Job drawing, mm, ordinate dimensions from the low corner. One solid piece. A direction names the side the tool comes from. Give positions to 0.01 mm unless a question says otherwise; leave off trailing zeros. Write each loop counter-clockwise with the first axis right and the second up, starting at its lowest first coordinate (ties: lowest second). Pieces come first, ordered by that corner, then holes. Notation, with made-up numbers: (7.25, -20) - (66.25, -20) arc R24 cw to (66.25, -8) - close; hole circle Ø3 at (55.5, -27). An arc over 180 degrees is marked (long way). Answer in a Markdown table with one row per item. Add a question column.
1. Band-saw the part on A-A on x = 8. Write the cut outline in (y, z), plus the area to 3 significant figures.
2. Probe line 1 along X through (y, z) = (95, 67); line 2 along Z through (x, y) = (52.5, 42); line 3 along Y through (x, z) = (47, 58). List the from-to ranges inside material, lowest first.
3. Band-saw the part on D-D on y = 95. Write the cut outline in (x, z), plus the area to 3 significant figures.
4. Which spindle directions (+Z, -Z, +X, -X, +Y, -Y) get a long thin tool onto all of the face, cutting with end or side? Do the marked faces 4, 5 and 6. Say none if no direction does.
5. Band-saw the part on C-C on x = 89. Write the cut outline in (y, z).
6. Drop flat-ended pins along their axis: pin 1 Ø1 at (x, z) = (46.5, 14) entering from +Y; pin 2 Ø0.8 at (y, z) = (17, 0.5) entering from -X; pin 3 Ø10 at (y, z) = (65.5, 10) entering from -X. Give the stop position or say it passes through.
7. Band-saw the part on B-B on y = 81.5. Write the cut outline in (x, z).
8. Pull direction Y, two halves, no side cores. Call the marked faces 1, 2 and 3: released by +Y, released by -Y, zero draft, split by the parting line, or undercut.
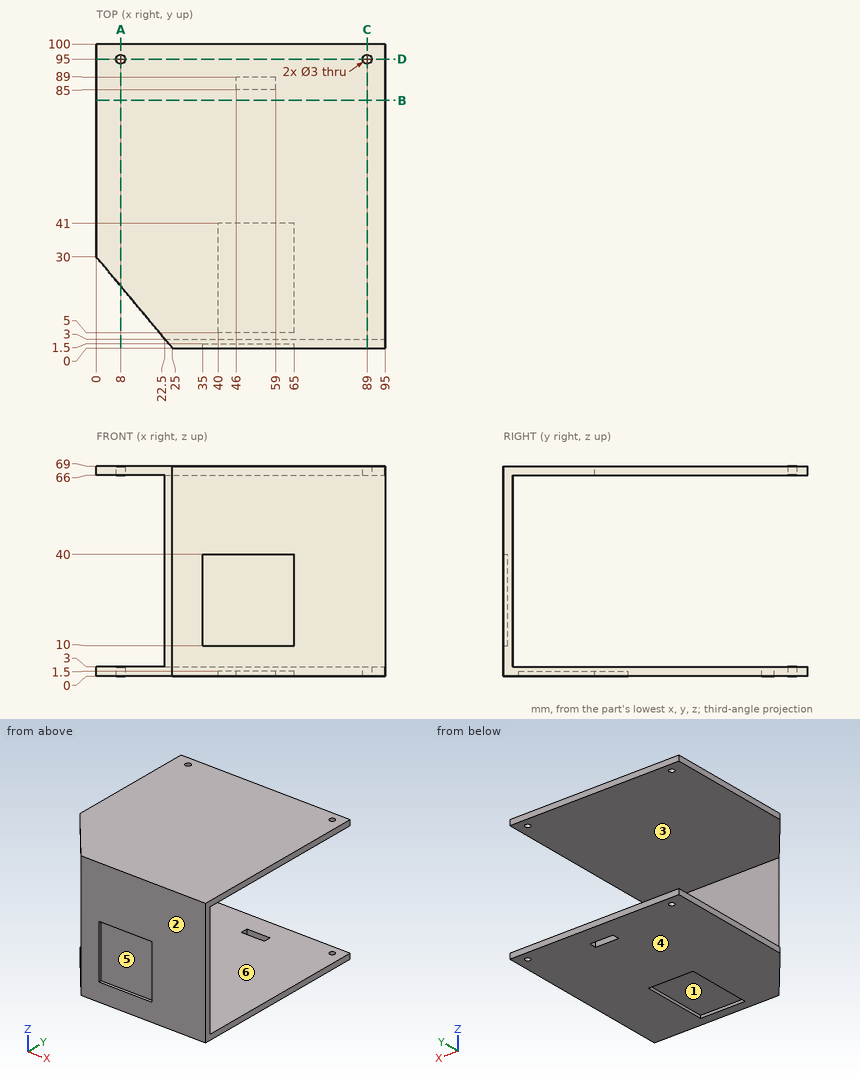
Values:
| question | item | result |
|---|---|---|
| 1 | outline | (20.4, 0) - (93.5, 0) - (93.5, 3) - (20.4, 3) - close; (20.4, 66) - (93.5, 66) - (93.5, 69) - (20.4, 69) - close; (96.5, 0) - (100, 0) - (100, 3) - (96.5, 3) - close; (96.5, 66) - (100, 66) - (100, 69) - (96.5, 69) - close |
| 1 | area | 460 mm² |
| 2 | line 1 | x = 0 to 6.5, 9.5 to 87.5, 90.5 to 95 |
| 2 | line 2 | z = 0 to 3, 66 to 69 |
| 2 | line 3 | y = 0 to 3 |
| 3 | outline | (0, 0) - (6.5, 0) - (6.5, 3) - (0, 3) - close; (0, 66) - (6.5, 66) - (6.5, 69) - (0, 69) - close; (9.5, 0) - (87.5, 0) - (87.5, 3) - (9.5, 3) - close; (9.5, 66) - (87.5, 66) - (87.5, 69) - (9.5, 69) - close; (90.5, 0) - (95, 0) - (95, 3) - (90.5, 3) - close; (90.5, 66) - (95, 66) - (95, 69) - (90.5, 69) - close |
| 3 | area | 534 mm² |
| 4 | face 4 | -Z, +X, -X, +Y, -Y |
| 4 | face 5 | -Y |
| 4 | face 6 | +X, -X, +Y |
| 5 | outline | (0, 0) - (93.5, 0) - (93.5, 3) - (3, 3) - (3, 66) - (93.5, 66) - (93.5, 69) - (0, 69) - close; (96.5, 0) - (100, 0) - (100, 3) - (96.5, 3) - close; (96.5, 66) - (100, 66) - (100, 69) - (96.5, 69) - close |
| 6 | pin 1 | stops at y = 3 |
| 6 | pin 2 | stops at x = 10.5 |
| 6 | pin 3 | passes through |
| 7 | outline | (0, 0) - (95, 0) - (95, 3) - (0, 3) - close; (0, 66) - (95, 66) - (95, 69) - (0, 69) - close |
| 8 | face 1 | undercut |
| 8 | face 2 | released by -Y |
| 8 | face 3 | zero draft |
